The listing builds one solid part. Answer for the finished solid, in the listing's coordinates (mm). Face numbers are marked on the shaded views. A direction names the side the tool comes from. Round coordinates to 2 decimals unless told otherwise and drop trailing zeros. Write each loop counter-clockwise with the first axis right and the second up, starting at its lowest first coordinate (ties: lowest second). Pieces come first, ordered by that corner, then holes.
from build123d import *

# Parameters (mm, degrees)
SKETCH2_W           = 56.4
SKETCH2_H           = 56.4
BOSS_EXTRUDE1_DEPTH = 76
SKETCH3_R           = 3.175
CUT_EXTRUDE1_DEPTH  = 76
CUT_EXTRUDE2_START  = -71
SKETCH5_R           = 2
CUT_EXTRUDE2_DEPTH  = 71
FILLET1_R           = 2
BOSS_EXTRUDE2_START = 2.5
SKETCH6_R           = 10
SKETCH6_R_2         = 3.175
BOSS_EXTRUDE2_DEPTH = 2.5
FILLET2_R           = 2


with BuildPart() as part:
    # Sketch2 → Boss-Extrude1 (new body)
    with BuildSketch(Plane(origin=(0, 0, 0), x_dir=(1, 0, 0), z_dir=(0, 1, 0))):
        Rectangle(SKETCH2_W, SKETCH2_H)
    extrude(amount=BOSS_EXTRUDE1_DEPTH)

    # Sketch3 → Cut-Extrude1 (cut)
    with BuildSketch(Plane(origin=(0, 76, 0), x_dir=(1, 0, 0), z_dir=(0, 1, 0))):
        with BuildLine():
            Line((-23.55, 21.55), (-23.55, 23.55))
            Line((-23.55, 23.55), (-21.55, 23.55))
            ThreePointArc((-21.55, 23.55), (-24.964213562, 24.964213562), (-23.55, 21.55))
        make_face()
        with BuildLine():
            Line((-21.55, 23.55), (-23.55, 23.55))
            Line((-23.55, 23.55), (-23.55, 21.55))
            ThreePointArc((-23.55, 21.55), (-22.135786438, 22.135786438), (-21.55, 23.55))
        make_face()
        with BuildLine():
            ThreePointArc((25.55, 23.55), (23.55, 25.55), (21.55, 23.55))
            Line((21.55, 23.55), (23.55, 23.55))
            Line((23.55, 23.55), (23.55, 21.55))
            ThreePointArc((23.55, 21.55), (24.964213562, 22.135786438), (25.55, 23.55))
        make_face()
        with BuildLine():
            Line((23.55, 23.55), (21.55, 23.55))
            ThreePointArc((21.55, 23.55), (22.135786438, 22.135786438), (23.55, 21.55))
            Line((23.55, 21.55), (23.55, 23.55))
        make_face()
        with Locations(Location((0, 0, 0), (0, 0, 270))):
            Circle(SKETCH3_R)
        with BuildLine():
            ThreePointArc((-21.55, -23.55), (-22.135786438, -22.135786438), (-23.55, -21.55))
            Line((-23.55, -21.55), (-23.55, -23.55))
            Line((-23.55, -23.55), (-21.55, -23.55))
        make_face()
        with BuildLine():
            Line((-23.55, -23.55), (-23.55, -21.55))
            ThreePointArc((-23.55, -21.55), (-24.964213562, -24.964213562), (-21.55, -23.55))
            Line((-21.55, -23.55), (-23.55, -23.55))
        make_face()
        with BuildLine():
            ThreePointArc((25.55, -23.55), (24.964213562, -22.135786438), (23.55, -21.55))
            Line((23.55, -21.55), (23.55, -23.55))
            Line((23.55, -23.55), (21.55, -23.55))
            ThreePointArc((21.55, -23.55), (23.55, -25.55), (25.55, -23.55))
        make_face()
        with BuildLine():
            Line((23.55, -23.55), (23.55, -21.55))
            ThreePointArc((23.55, -21.55), (22.135786438, -22.135786438), (21.55, -23.55))
            Line((21.55, -23.55), (23.55, -23.55))
        make_face()
    extrude(amount=-CUT_EXTRUDE1_DEPTH, mode=Mode.SUBTRACT)

    # Sketch5 → Cut-Extrude2 (cut)
    # profile 1 of 4: a face of its own
    with BuildSketch(Plane(origin=(0, 0, 0), x_dir=(-1, 0, 0), z_dir=(0, -1, 0)).offset(CUT_EXTRUDE2_START)):
        with BuildLine():
            Line((19.05, 28.2), (19.05, 21.05))
            ThreePointArc((19.05, 21.05), (19.635786438, 19.635786438), (21.05, 19.05))
            Line((21.05, 19.05), (28.2, 19.05))
            Line((28.2, 19.05), (28.2, 28.2))
            Line((28.2, 28.2), (19.05, 28.2))
        make_face()
        with Locations((23.55, 23.55)):
            Circle(SKETCH5_R, mode=Mode.SUBTRACT)
    # profile 2 of 4: a face of its own
    with BuildSketch(Plane(origin=(0, 0, 0), x_dir=(-1, 0, 0), z_dir=(0, -1, 0)).offset(CUT_EXTRUDE2_START)):
        with BuildLine():
            Line((-19.05, 21.05), (-19.05, 28.2))
            Line((-19.05, 28.2), (-28.2, 28.2))
            Line((-28.2, 28.2), (-28.2, 19.05))
            Line((-28.2, 19.05), (-21.05, 19.05))
            ThreePointArc((-21.05, 19.05), (-19.635786438, 19.635786438), (-19.05, 21.05))
        make_face()
        with Locations((-23.55, 23.55)):
            Circle(SKETCH5_R, mode=Mode.SUBTRACT)
    # profile 3 of 4: a face of its own
    with BuildSketch(Plane(origin=(0, 0, 0), x_dir=(-1, 0, 0), z_dir=(0, -1, 0)).offset(CUT_EXTRUDE2_START)):
        with BuildLine():
            Line((28.2, -28.2), (28.2, -19.05))
            Line((28.2, -19.05), (21.05, -19.05))
            ThreePointArc((21.05, -19.05), (19.635786438, -19.635786438), (19.05, -21.05))
            Line((19.05, -21.05), (19.05, -28.2))
            Line((19.05, -28.2), (28.2, -28.2))
        make_face()
        with Locations((23.55, -23.55)):
            Circle(SKETCH5_R, mode=Mode.SUBTRACT)
    # profile 4 of 4: a face of its own
    with BuildSketch(Plane(origin=(0, 0, 0), x_dir=(-1, 0, 0), z_dir=(0, -1, 0)).offset(CUT_EXTRUDE2_START)):
        with BuildLine():
            Line((-21.05, -19.05), (-28.2, -19.05))
            Line((-28.2, -19.05), (-28.2, -28.2))
            Line((-28.2, -28.2), (-19.05, -28.2))
            Line((-19.05, -28.2), (-19.05, -21.05))
            ThreePointArc((-19.05, -21.05), (-19.635786438, -19.635786438), (-21.05, -19.05))
        make_face()
        with Locations((-23.55, -23.55)):
            Circle(SKETCH5_R, mode=Mode.SUBTRACT)
    extrude(amount=CUT_EXTRUDE2_DEPTH, mode=Mode.SUBTRACT)

    # Fillet1
    fillet1_edges = [part.edges().sort_by_distance(p)[0] for p in [
        (-19.05, 35.5, -28.2),
        (-28.2, 35.5, -19.05),
        (28.2, 35.5, -19.05),
        (19.05, 35.5, -28.2),
        (19.05, 35.5, 28.2),
        (28.2, 35.5, 19.05),
        (-28.2, 35.5, 19.05),
        (-19.05, 35.5, 28.2),
    ]]
    fillet(fillet1_edges, radius=FILLET1_R)

    # Sketch6 → Boss-Extrude2 (add)
    with BuildSketch(Plane(origin=(0, 76, 0), x_dir=(1, 0, 0), z_dir=(0, 1, 0)).offset(BOSS_EXTRUDE2_START)):
        with Locations(Location((0, 0, 0), (0, 0, 270))):
            Circle(SKETCH6_R)
        with Locations(Location((0, 0, 0), (0, 0, 270))):
            Circle(SKETCH6_R_2, mode=Mode.SUBTRACT)
    extrude(amount=-BOSS_EXTRUDE2_DEPTH)

    # Fillet2
    fillet2_edges = [part.edges().sort_by_distance(p)[0] for p in [
        (0, 78.5, -10),
    ]]
    fillet(fillet2_edges, radius=FILLET2_R)


solid = part.part
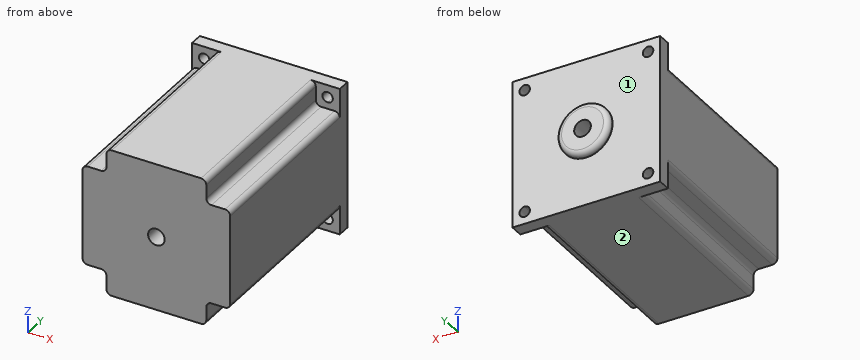
1. Section A-A on z = 0 is taken. Determine the outline of the cut face in (x, y) (3 decimals), plus the area to 3 significant figures.
Geometry says:
outline: (-28.2, 0) - (-3.175, 0) - (-3.175, 78.5) - (-8, 78.5) arc R2 ccw to (-10, 76.5) - (-10, 76) - (-28.2, 76) - close; (3.175, 0) - (28.2, 0) - (28.2, 76) - (10, 76) - (10, 76.5) arc R2 ccw to (8, 78.5) - (3.175, 78.5) - close
area: 3,840 mm2
2. Section B-B on y = 54 is taken. Determine the outline of the cut face in (x, z) (3 decimals).
Geometry says:
outline: (-28.2, -17.05) arc R2 ccw to (-26.2, -19.05) - (-21.05, -19.05) arc R2 cw to (-19.05, -21.05) - (-19.05, -26.2) arc R2 ccw to (-17.05, -28.2) - (17.05, -28.2) arc R2 ccw to (19.05, -26.2) - (19.05, -21.05) arc R2 cw to (21.05, -19.05) - (26.2, -19.05) arc R2 ccw to (28.2, -17.05) - (28.2, 17.05) arc R2 ccw to (26.2, 19.05) - (21.05, 19.05) arc R2 cw to (19.05, 21.05) - (19.05, 26.2) arc R2 ccw to (17.05, 28.2) - (-17.05, 28.2) arc R2 ccw to (-19.05, 26.2) - (-19.05, 21.05) arc R2 cw to (-21.05, 19.05) - (-26.2, 19.05) arc R2 ccw to (-28.2, 17.05) - close; hole circle Ø6.35 at (0, 0)
3. Section C-C on x = 24.5 is taken. Determine the outline of the cut face in (y, z).
Geometry says:
outline: (0, -19.05) - (71, -19.05) - (71, -21.79) - (76, -21.79) - (76, 21.79) - (71, 21.79) - (71, 19.05) - (0, 19.05) - close; (71, -28.2) - (76, -28.2) - (76, -25.31) - (71, -25.31) - close; (71, 25.31) - (76, 25.31) - (76, 28.2) - (71, 28.2) - close
4. Given pin 1 (9 mm diameter, centred on x = -21, z = 22, fed in from -Y); pin 2 (9 mm diameter, centred on x = 25, z = 25, fed in from -Y); pin 3 (1.5 mm diameter, centred on y = 53, z = -24, fed in from +X); pin 4 (2.5 mm diameter, centred on x = -22.5, y = 18.5, fed in from -Z), each flat-ended and moving along its own axis, determine where each tip first touches the part or whether it passes through.
Geometry says:
pin 1: stops at y = 0
pin 2: stops at y = 71
pin 3: stops at x = 19.05
pin 4: stops at z = -19.05
5. Straight lines are drawn through the part: line 1 along X through (y, z) = (74.2, 23.55); line 2 along X through (y, z) = (51, -1.5). For each, find the intervals that lie inside material, in ascending order.
Geometry says:
line 1: x = -28.2 to -25.55, -21.55 to 21.55, 25.55 to 28.2
line 2: x = -28.2 to -2.8, 2.8 to 28.2
6. Section D-D on x = -18 is taken. Determine the outline of the cut face in (y, z), plus the area to 3 significant figures.
Geometry says:
outline: (0, -27.96) - (71, -27.96) - (71, -28.2) - (76, -28.2) - (76, 28.2) - (71, 28.2) - (71, 27.96) - (0, 27.96) - close
area: 4,250 mm2
7. A tool of negligible diameter and unlimited length cuts with its end or side. For the marked faces 1 and 2, from which of +Z, -Z, +X, -X, +Y, -Y can it reach the whole face along a straight path? Write none if from no direction.
Geometry says:
face 1: +Y
face 2: -Z, +X, -X, +Y, -Y
